Geometry: final body of the model. Coordinates: model frame, mm. Give positions to 0.01 mm unless a question says otherwise; leave off trailing zeros. Order: outer loops, then holes, each group sorted by start corner. A loop starts at its lowest first (then second) coordinate and runs counter-clockwise, first axis right, second up. Notation, with made-up numbers: (27, 34.25) -> (67, 34.25) arc R26 ccw to (67, 51.25) -> close; hole circle Ø8 at (-8.5, 9.25). An arc over 180 degrees is marked (long way). Answer in a Markdown table with one row per item. Add a question column.
Q1. Cut plane A-A on z = 0. Return the cut outline in (x, y).
Q2. Cut plane B-B on y = 1.5. Return the cut outline in (x, z).
Q3. Cut plane D-D on y = 4.75. Return the cut outline in (x, z), and give its area (3 significant figures).
Q4. Line query: line 1 along X through (y, z) = (-10.5, 0); line 2 along Z through (x, y) = (0.25, 5.5). Output: solid intervals per line, ascending. Write a range as from..to.
Q5. Pull-direction query (Z, two-part tool) for faces 1 (the face through (4, -14, 4)), 2 (the face through (5, -6.9, 1.6)), 3 (the face through (3.35, -6.9, -6.43)); classes: +Z half, -Z half, draft (parallel to the pull), parting line (faces both ways), or undercut.
Q6. Cut plane C-C on y = -9. Return the cut outline in (x, z).
Q7. Contact query for flat-ended pins moving along their axis: P1, Ø4, axis at y = 4.5, z = 6.5, coming from the -X side; P2, Ø10, axis at x = -3.5, y = -12, coming from the -Z side; P3, Ø8, axis at x = -7.5, z = 6.5, coming from the -Y side; P4, Ø3, axis at x = 7, y = 0.5, coming from the -Z side. Output: stop coordinate, or through.
from build123d import *

# Parameters (mm, degrees)
CROQUIS3_R              = 7.25
CROQUIS3_R_2            = 5.25
SALIENTE_EXTRUIR1_DEPTH = 14
CROQUIS4_W              = 14.959615834
CROQUIS4_H              = 3.245468311
CORTAR_EXTRUIR1_DEPTH   = 10


with BuildPart() as part:
    # Croquis2 → Revolución1 (revolve)
    with BuildSketch(Plane.XY):
        Polygon((-5.25, 0), (-8, 7.5), (-10, 7.5), (-7.25, 0), align=None)
    revolve(axis=Axis((0, 7.5, 0), (0, -1, 0)))

    # Croquis3 → Saliente-Extruir1 (add)
    with BuildSketch(Plane.XZ):
        Circle(CROQUIS3_R)
        Circle(CROQUIS3_R_2, mode=Mode.SUBTRACT)
    extrude(amount=SALIENTE_EXTRUIR1_DEPTH)

    # Croquis4 → Cortar-Extruir1 (cut)
    with BuildSketch(Plane(origin=(0, 7.5, 0), x_dir=(1, 0, 0), z_dir=(0, 1, 0))):
        with Locations((0, 9.622734156)):
            Rectangle(CROQUIS4_W, CROQUIS4_H)
    extrude(amount=-CORTAR_EXTRUIR1_DEPTH, mode=Mode.SUBTRACT)


solid = part.part
Completed:
| question | item | result |
|---|---|---|
| 1 | outline | (-10, 7.5) -> (-7.25, 0) -> (-7.25, -14) -> (-5.25, -14) -> (-5.25, 0) -> (-8, 7.5) -> close; (5.25, -14) -> (7.25, -14) -> (7.25, 0) -> (10, 7.5) -> (8, 7.5) -> (5.25, 0) -> close |
| 2 | outline | circle Ø15.6 at (0, 0); hole circle Ø11.6 at (0, 0) |
| 3 | outline | (-4.1, -8) -> (4.1, -8) arc R8.99 ccw (long way) to start; hole circle Ø13.98 at (0, 0) |
| 3 | area | 94.9 mm² |
| 4 | line 1 | x = -7.25..-5.25, 5.25..7.25 |
| 4 | line 2 | z = -8..-7.26, 7.26..9.26 |
| 5 | face 1 | draft |
| 5 | face 2 | undercut |
| 5 | face 3 | parting line |
| 6 | outline | circle Ø14.5 at (0, 0); hole circle Ø10.5 at (0, 0) |
| 7 | P1 | stops at x = -7.95 |
| 7 | P2 | stops at z = -7.25 |
| 7 | P3 | stops at y = -14 |
| 7 | P4 | stops at z = -5.19 |
